```python
from build123d import *

# Parameters (mm, degrees)
CROQUIS1_W              = 1370
CROQUIS1_H              = 76.2
SALIENTE_EXTRUIR1_DEPTH = 76.2
SALIENTE_EXTRUIR2_DEPTH = 76.2


with BuildPart() as part:
    # Croquis1 → Saliente-Extruir1 (new body)
    with BuildSketch(Plane.XY):
        with Locations((685, 38.1)):
            Rectangle(CROQUIS1_W, CROQUIS1_H)
    extrude(amount=SALIENTE_EXTRUIR1_DEPTH)

    # Croquis2 → Saliente-Extruir2 (add)
    with BuildSketch(Plane.XY.offset(76.2)):
        Polygon((723.1, 1845.423164628), (723.1, 1622.629269336), (1285.954223436, 76.2), (1367.044569699, 76.2), align=None)
        Polygon((2.955430301, 76.2), (84.045776564, 76.2), (646.9, 1622.629269336), (646.9, 1845.423164628), align=None)
    extrude(amount=-SALIENTE_EXTRUIR2_DEPTH)


solid = part.part
```
Geometry: final body of the model. Coordinates: model frame, mm. A direction names the side the tool comes from. Coordinates: 2 decimals unless noted, no trailing zeros. Order: outer loops, then holes, each group sorted by start corner. A loop starts at its lowest first (then second) coordinate and runs counter-clockwise, first axis right, second up. Notation, with made-up numbers: (15, -11.5) - (58, -11.5) arc R22 ccw to (58, 16.5) - close; hole circle Ø7 at (59.5, 13.5). An arc over 180 degrees is marked (long way). Return JSON: item names as keys, results as strings. Group by question number.
1. Pull-direction query (Y, two-part tool) for faces 4 (the face through (675, 0, 38)), 5 (the face through (377, 927, 0)), 6 (the face through (677, 76.2, 38)); classes: pulls with the +Y half, pulls with the -Y half, needs draft (parallel to the pull), parting line crosses it, or undercut.
2. Cut plane B-B (y = 1735). Output: boundary loops of the cut face in (x, z).
3. Material intervals for line 1 along X through (y, z) = (542, 25); line 2 along Y through (x, z) = (714, 42.5); line 3 along X through (y, z) = (899, 5), sorted ascending. Write a range as [from, to].
4. Set-up query: faces 1 (the face through (1049.58, 948.43, 38.63)), 2 (the face through (1000.6, 860.2, 38.6)), 3 (the face through (646.9, 1732, 39)). Return all of +Z, -Z, +X, -X, +Y, -Y with unobstructed straight access to the full face (end or side cutting, diameter ignored); none if empty.
5. Pin query (flat end, axial travel): pin 1 (10 mm diameter, centred on y = 909.5, z = 61, fed in from -X); pin 2 (4 mm diameter, centred on y = 1608.5, z = 17, fed in from -X); pin 3 (23 mm diameter, centred on y = 1787.5, z = 50, fed in from +X). Return the tip coordinate at first contact, or that it passes through.
6. Cut plane A-A (x = 201.5). Output: boundary loops of the cut face in (y, z), plus the area to 3 significant figures.
7. Cut plane C-C (z = 45.5). Output: boundary loops of the cut face in (x, y), plus the area to 3 significant figures.
Resolved:
{
 "1": {"face 4": "pulls with the -Y half", "face 5": "needs draft", "face 6": "undercut"},
 "2": {"outline": "(606.71, 0) - (646.9, 0) - (646.9, 76.2) - (606.71, 76.2) - close; (723.1, 0) - (763.29, 0) - (763.29, 76.2) - (723.1, 76.2) - close"},
 "3": {"line 1": "x = [172.49, 253.58], [1116.42, 1197.51]", "line 2": "y = [0, 76.2]", "line 3": "x = [302.43, 383.52], [986.48, 1067.57]"},
 "4": {"face 1": "+Z, -Z, +X, +Y", "face 2": "+Z, -Z", "face 3": "+Z, -Z, +Y"},
 "5": {"pin 1": "stops at x = 304.43", "pin 2": "stops at x = 559.94", "pin 3": "stops at x = 748.37"},
 "6": {"outline": "(0, 0) - (76.2, 0) - (76.2, 76.2) - (0, 76.2) - close; (398.9, 0) - (621.7, 0) - (621.7, 76.2) - (398.9, 76.2) - close", "area": "22,800 mm²"},
 "7": {"outline": "(0, 0) - (1370, 0) - (1370, 76.2) - (1367.04, 76.2) - (723.1, 1845.42) - (723.1, 1622.63) - (1285.95, 76.2) - (84.05, 76.2) - (646.9, 1622.63) - (646.9, 1845.42) - (2.96, 76.2) - (0, 76.2) - close", "area": "373,000 mm²"}
}
